from build123d import *

# Parameters (mm, degrees)
SKETCH1_W           = 30
SKETCH1_H           = 55
BOSS_EXTRUDE1_DEPTH = 3
SKETCH2_W           = 7
SKETCH2_H           = 7
BOSS_EXTRUDE2_DEPTH = 2
SKETCH3_R           = 1.5
CUT_EXTRUDE1_DEPTH  = 2
SKETCH4_R           = 2.5
CUT_EXTRUDE2_DEPTH  = 1
FILLET2_R           = 0.5


with BuildPart() as part:
    # Sketch1 → Boss-Extrude1 (new body)
    with BuildSketch(Plane(origin=(0, 0, 0), x_dir=(1, 0, 0), z_dir=(0, 1, 0))):
        Rectangle(SKETCH1_W, SKETCH1_H)
    extrude(amount=BOSS_EXTRUDE1_DEPTH)

    # Sketch2 → Boss-Extrude2 (add)
    with BuildSketch(Plane(origin=(0, 3, 0), x_dir=(1, 0, 0), z_dir=(0, 1, 0))):
        with Locations((-18, 0)):
            Rectangle(SKETCH2_W, SKETCH2_H)
    extrude(amount=-BOSS_EXTRUDE2_DEPTH)

    # Sketch3 → Cut-Extrude1 (cut)
    with BuildSketch(Plane(origin=(0, 3, 0), x_dir=(1, 0, 0), z_dir=(0, 1, 0))):
        with Locations(Location((-18, 0, 0), (0, 0, 270))):
            Circle(SKETCH3_R)
    extrude(amount=-CUT_EXTRUDE1_DEPTH, mode=Mode.SUBTRACT)

    # Sketch4 → Cut-Extrude2 (cut)
    with BuildSketch(Plane(origin=(0, 3, 0), x_dir=(1, 0, 0), z_dir=(0, 1, 0))):
        with Locations(Location((-18, 0, 0), (0, 0, 270))):
            Circle(SKETCH4_R)
    extrude(amount=-CUT_EXTRUDE2_DEPTH, mode=Mode.SUBTRACT)

    # Fillet2
    fillet2_edges = [part.edges().sort_by_distance(p)[0] for p in [
        (15, 3, 0),
        (-15, 3, 15.5),
        (-18.25, 3, 3.5),
        (0, 3, -27.5),
        (-18.25, 3, -3.5),
        (-21.5, 3, 0),
        (-18, 3, -2.5),
        (-18, 2, -2.5),
        (-18, 2, -1.5),
        (-15, 3, -15.5),
        (0, 3, 27.5),
    ]]
    fillet(fillet2_edges, radius=FILLET2_R - 0.0001)  # a hair under: the kernel refuses the full size


solid = part.part
Here's how the part is built. I have some questions about the finished solid (model axes, mm). A direction names the side the tool comes from. Coordinates: 2 decimals unless noted, no trailing zeros. Write each loop counter-clockwise with the first axis right and the second up, starting at its lowest first coordinate (ties: lowest second). Pieces come first, ordered by that corner, then holes.
1) If we section it at C-C (z = -5.5): List the corners of the cut face in (x, y) for me, plus the area to 3 significant figures.
Filled in:
outline: (-15, 0) - (15, 0) - (15, 2.5) arc R0.5 ccw to (14.5, 3) - (-14.5, 3) arc R0.5 ccw to (-15, 2.5) - close
area: 89.9 mm2
2) I'm going to push flat-ended pins straight in: pin 1 (0.8 mm diameter, centred on y = 1, z = 5, fed in from -X); pin 2 (4.5 mm diameter, centred on x = -18, z = 0, fed in from -Y); pin 3 (1.7 mm diameter, centred on x = -19, y = 2, fed in from -Z). Where does each tip first touch, or does it pass through?
Filled in:
pin 1: stops at x = -15
pin 2: stops at y = 1
pin 3: stops at z = -3.5
3) Thinking about a two-plate mould opening in Z: for faces 1 (the face through (0, 0, 0)), 2 (the face through (0, 1, 27.5)), 3 (the face through (-16.735, 1.254, 0.806)), which applies, +Z half, -Z half, draft (parallel to the pull), parting line (faces both ways), or undercut?
Filled in:
face 1: draft
face 2: +Z half
face 3: undercut
4) Which directions (+Z, -Z, +X, -X, +Y, -Y) give clear straight access to the entire face, cutting with the end or side of a thin tool? Please do faces 4 (the face through (-18, 2, -3.5)), 5 (the face through (-18, 2, 3.5)), 6 (the face through (-20, 1, 0)).
Filled in:
face 4: -Z, -X, +Y, -Y
face 5: +Z, -X, +Y, -Y
face 6: +Z, -Z, -X, -Y
5) If I drill on line 1 (X direction, y = 2.5, z = 0); line 2 (X direction, y = 2.6, z = -9); line 3 (Z direction, x = -20, y = 1.2), over which ranges is the centre line in solid material (lowest first)?
Filled in:
line 1: x = -21.5 to -20.5, -15.5 to 15
line 2: x = -14.99 to 14.99
line 3: z = -3.5 to 3.5
